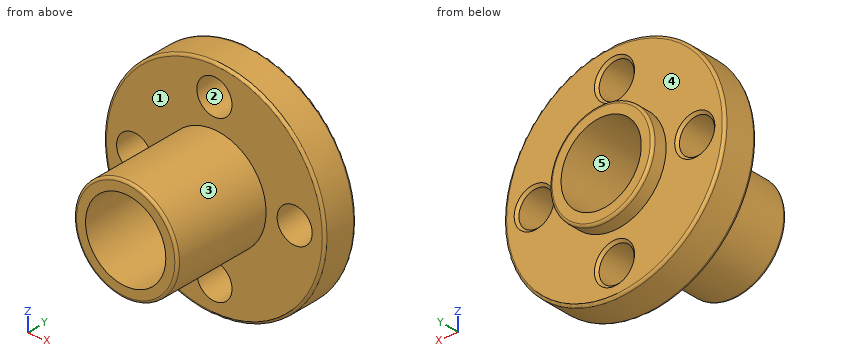
Autodesk Inventor part; units mm, degrees
ref_plane "YZ Plane" through (0, 0, 0) normal (1, 0, 0) x (0, 1, 0)
ref_plane "XZ Plane" through (0, 0, 0) normal (0, 1, 0) x (-1, 0, 0)
ref_plane "XY Plane" through (0, 0, 0) normal (0, 0, 1) x (1, 0, 0)
sketch "Sketch1" plane through (0, 0, 0) normal (0, 0, 1) x (1, 0, 0)
  line L0 (4, 7.5) -> (4, -7.5)
  line L1 (4, -7.5) -> (5.15, -7.5)
  line L2 (5.15, -7.5) -> (5.15, 2.5)
  line L3 (5.15, 2.5) -> (11, 2.5)
  line L4 (11, 2.5) -> (11, 6)
  line L5 (11, 6) -> (5.15, 6)
  line L6 (5.15, 6) -> (5.15, 7.5)
  line L7 (5.15, 7.5) -> (4, 7.5)
  line L8 (0, 0) -> (22.0974, 0) construction
  line L9 (0, -10.5) -> (0, 10.5)
  dimension "d1" = 3.5
  dimension "d2" = 1.5
  dimension "d3" = 15
  dimension "d4" = 11
  dimension "d5" = 4
  dimension "d6" = 5.15
revolve "Revolution1" add sketch "Sketch1" angle 360 about axis through (0, -10, 0) along (0, 1, 0)
sketch "Sketch2" plane through (0, 6, 0) normal (0, 1, 0) x (1, 0, 0)
  circle A0 centre (0, 0) radius 8 construction
  line L0 (8, 0) -> (-8, 0) construction
  line L1 (0, -8) -> (0, 8) construction
  circle A1 centre (-8, 0) radius 1.75
  circle A2 centre (0, 8) radius 1.75
  circle A3 centre (8, 0) radius 1.75
  circle A4 centre (0, -8) radius 1.75
  dimension "d8" = 16
  dimension "d9" = 3.5
extrude "Extrusion1" cut sketch "Sketch2" against normal through all
chamfer "Chamfer1" distance 0.25 angle 45 4 edges at (-1.75, 6, 8) (6.25, 6, 0) (-1.75, 6, -8) (-9.75, 6, 0)
fillet "Fillet1" radius 0.25 4 edges at (-11, 6, 0) (-11, 2.5, 0) (-5.15, 7.5, 0) (-5.15, -7.5, 0)
thread "Thread1"
properties part number "TR8 Leadscrew Nut" material "Brass, Soft Yellow"
The listing builds one solid part. Answer for the finished solid, in the listing's coordinates (mm). Face numbers are marked on the shaded views. A direction names the side the tool comes from. Round coordinates to 2 decimals unless told otherwise and drop trailing zeros. Order: outer loops, then holes, each group sorted by start corner. A loop starts at its lowest first (then second) coordinate and runs counter-clockwise, first axis right, second up. Notation, with made-up numbers: M -21,15 L 30,15 A30 ccw 30,40 Z; hole C 51,57.25 d4. An arc over 180 degrees is marked long. Answer in a Markdown table with one row per item. Add a question column.
1) Consider line 1 along X through (y, z) = (3.8, 0); line 2 along Z through (x, y) = (0, 0.75). Determine where each line is inside the solid, lowest interval first. Write a range as from..to.
2) Flat-ended cylindrical pins translate along their axes: pin 1 Ø5.5 at (x, z) = (-8, 0) entering from +Y; pin 2 Ø10 at (x, z) = (-3.5, 5) entering from -Y; pin 3 Ø4.5 at (x, z) = (0, 8) entering from -Y; pin 4 Ø1 at (y, z) = (-2.5, -2) entering from -X. Find the tip coordinate at first contact, or state that the pin passes through.
3) Which of the six approach directions +Z, -Z, +X, -X, +Y, -Y give full straight-line access (tool end or side, diameter ignored) to the marked faces 4 and 5?
4) Determine the mould class of the marked faces 1, 2 and 3 for opening direction X: pulls with the +X half, pulls with the -X half, needs draft (parallel to the pull), parting line crosses it, or undercut.
5) The part is cut by section D-D on y = 5.25. Determine the outline of the cut face in (x, z), plus the area to 3 significant figures.
6) The part is cut by section B-B on x = 0. Count the separate pieces of the cut face and the enclosed holes in it, plus the area to 3 significant figures.
7) The part is cut by section A-A on y = -4.75. Determine the outline of the cut face in (x, z), plus the area to 3 significant figures.
Findings below:
| question | item | result |
|---|---|---|
| 1 | line 1 | x = -11..-9.75, -6.25..-4, 4..6.25, 9.75..11 |
| 1 | line 2 | z = -5.15..-4, 4..5.15 |
| 2 | pin 1 | stops at y = 6 |
| 2 | pin 2 | stops at y = -7.5 |
| 2 | pin 3 | stops at y = 2.5 |
| 2 | pin 4 | stops at x = -4.93 |
| 3 | face 4 | +Y |
| 3 | face 5 | +Y, -Y |
| 4 | face 1 | needs draft |
| 4 | face 2 | undercut |
| 4 | face 3 | parting line crosses it |
| 5 | outline | C 0,0 d22; hole C -8,0 d3.5; hole C 0,0 d8; hole C 0,-8 d3.5; hole C 0,8 d3.5; hole C 8,0 d3.5 |
| 5 | area | 291 mm² |
| 6 | separate pieces | 4 |
| 6 | enclosed holes | 0 |
| 6 | area | 50.7 mm² |
| 7 | outline | C 0,0 d10.3; hole C 0,0 d8 |
| 7 | area | 33.1 mm² |
